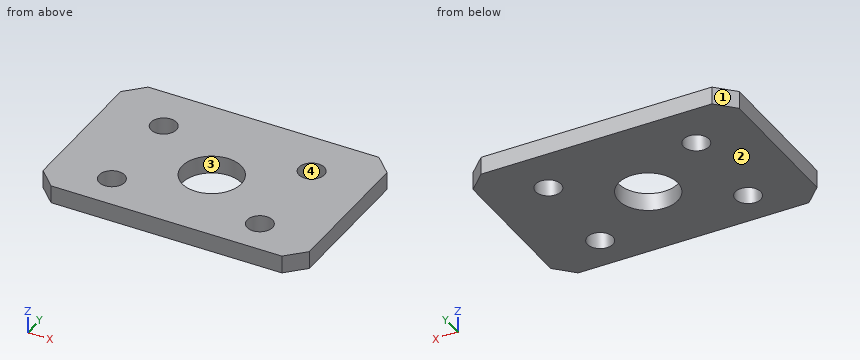
```python
from build123d import *

# Parameters (mm, degrees)
SKETCH_1_W               = 33
SKETCH_1_H               = 47
SKETCH_1_R               = 5
EXTRUDE_1_DEPTH          = 4
EXTRUDE_2_DEPTH          = 30
SKETCH_4_W               = 33
SKETCH_4_H               = 38
EXTRUDE_3_DEPTH          = 4
CHAMFER_1_SIZE           = 3
SKETCH_5_W               = 10
SKETCH_5_H               = 30
EXTRUDE_4_DEPTH          = 6
SKETCH_6_R               = 2.15
CUT_EXTRUDE_1_DEPTH      = 88.143559716
SKETCH_7_R               = 2.15
CUT_EXTRUDE_2_DEPTH      = 60
SKETCH_8_W               = 142.872393379
SKETCH_8_H               = 129.651084076
CUT_EXTRUDE_3_DEPTH      = 88.143559716
CUT_EXTRUDE_START        = -26
SKETCH_9_W               = 6
SKETCH_9_H               = 85
SKETCH_9_H_2             = 55
CUT_EXTRUDE_4_DEPTH      = 26
SKETCH_10_R              = 6.65
EXTRUDE_5_DEPTH          = 5.2
EXTRUDE_6_DEPTH          = 6
CHAMFER_2_SIZE           = 5.2
EXTRUDE_START            = -6
SKETCH_12_R              = 2.15
EXTRUDE_7_DEPTH          = 6
SKETCH_13_R              = 2.15
CUT_EXTRUDE_5_DEPTH      = 110.424128966
CUT_EXTRUDE_6_DEPTH      = 110.424128966
CUT_EXTRUDE_6_DEPTH_BACK = 110.424128966
SKETCH_14_W              = 45
SKETCH_14_H              = 81.938700875
SKETCH_15_W              = 48.923705392
SKETCH_15_H              = 34.943280138
CUT_EXTRUDE_7_DEPTH      = 6.2
CHAMFER_3_SIZE           = 3


with BuildPart() as part:
    # 草图1 → 凸台-拉伸1 (new body)
    with BuildSketch(Plane.XY):
        with Locations((16.5, 23.5)):
            Rectangle(SKETCH_1_W, SKETCH_1_H)
        with Locations((16.5, 31)):
            Circle(SKETCH_1_R, mode=Mode.SUBTRACT)
    extrude(amount=EXTRUDE_1_DEPTH)

    # 草图3 → 凸台-拉伸2 (add)
    with BuildSketch(Plane(origin=(0, 0, 0), x_dir=(-1, 0, 0), z_dir=(0, 0, -1))):
        Polygon((0, -38), (-33, -38), (-33, 47), (-39, 47), (-39, -63), (-26.75, -63), (-26.75, -43), (-6.25, -43), (-6.25, -63), (6, -63), (6, 47), (0, 47), align=None)
    extrude(amount=-EXTRUDE_2_DEPTH)

    # 草图4 → 凸台-拉伸3 (add)
    with BuildSketch(Plane(origin=(0, 0, 0), x_dir=(-1, 0, 0), z_dir=(0, 0, -1))):
        with Locations((-16.5, -19)):
            Rectangle(SKETCH_4_W, SKETCH_4_H)
    extrude(amount=-EXTRUDE_3_DEPTH)

    # 倒角1
    chamfer_1_edges = [part.edges().sort_by_distance(p)[0] for p in [
        (-6, 47, 15),
        (-6, -63, 15),
        (39, -63, 15),
        (39, 47, 15),
    ]]
    chamfer(chamfer_1_edges, length=CHAMFER_1_SIZE)

    # 草图5 → 凸台-拉伸4 (add)
    with BuildSketch(Plane(origin=(39, 0, 0), x_dir=(0, 0, -1), z_dir=(1, 0, 0))):
        with Locations((-35, -23)):
            Rectangle(SKETCH_5_W, SKETCH_5_H)
    extrude(amount=-EXTRUDE_4_DEPTH)

    # 草图6 → 切除-拉伸1 (cut, through all)
    with BuildSketch(Plane(origin=(39, 0, 0), x_dir=(0, 0, -1), z_dir=(1, 0, 0))):
        with Locations(Location((-11, -32, 0), (0, 0, 90))):
            Circle(SKETCH_6_R)
        with Locations(Location((-35, -32, 0), (0, 0, 90))):
            Circle(SKETCH_6_R)
        with Locations(Location((-11, -14, 0), (0, 0, 90))):
            Circle(SKETCH_6_R)
        with Locations(Location((-35, -14, 0), (0, 0, 90))):
            Circle(SKETCH_6_R)
    extrude(amount=-CUT_EXTRUDE_1_DEPTH, mode=Mode.SUBTRACT)

    # 草图7 → 切除-拉伸2 (cut)
    with BuildSketch(Plane.ZY.offset(6)):
        with Locations(Location((15, -53, 0), (0, 0, 270))):
            Circle(SKETCH_7_R)
    extrude(amount=-CUT_EXTRUDE_2_DEPTH, mode=Mode.SUBTRACT)

    # 镜向1: part across plane


with BuildPart() as part_1:
    add(part.part)
    add(part.part.mirror(Plane(origin=(39, 0, 0), x_dir=(0, 0, 1), z_dir=(1, 0, 0))))

    # 草图8 → 切除-拉伸3 (cut, through all)
    with BuildSketch(Plane(origin=(39, 0, 0), x_dir=(0, 0, -1), z_dir=(1, 0, 0))):
        with Locations((-14.281868294, -7.269848701)):
            Rectangle(SKETCH_8_W, SKETCH_8_H)
    extrude(amount=-CUT_EXTRUDE_3_DEPTH, mode=Mode.SUBTRACT)

    # 草图9 → 切除-拉伸4 (cut)
    with BuildSketch(Plane.XY.offset(30).offset(CUT_EXTRUDE_START)):
        with Locations((81, 4.5)):
            Rectangle(SKETCH_9_W, SKETCH_9_H)
        with Locations((42, 19.5)):
            Rectangle(SKETCH_9_W, SKETCH_9_H_2)
    extrude(amount=CUT_EXTRUDE_4_DEPTH, mode=Mode.SUBTRACT)

    # 草图10 → 凸台-拉伸5 (add)
    with BuildSketch(Plane.XY.offset(4)):
        Polygon((42, 47), (39, 44), (39, 17), (84, 17), (84, 44), (81, 47), align=None)
        with Locations((61.5, 31)):
            Circle(SKETCH_10_R, mode=Mode.SUBTRACT)
    extrude(amount=EXTRUDE_5_DEPTH)

    # 草图11 → 凸台-拉伸6 (add)
    with BuildSketch(Plane.ZY.offset(-39)):
        Polygon((40, -8), (4, -8), (4, 17), (9.2, 17), align=None)
    extrude(amount=-EXTRUDE_6_DEPTH)

    # 倒角2
    chamfer_2_edges = [part_1.edges().sort_by_distance(p)[0] for p in [
        (64.5, 17, 4),
    ]]
    chamfer(chamfer_2_edges, length=CHAMFER_2_SIZE - 0.0001)  # a hair under: the kernel refuses the full size

    # 草图12 → 凸台-拉伸7 (add)
    with BuildSketch(Plane(origin=(84, 0, 0), x_dir=(0, 0, -1), z_dir=(1, 0, 0)).offset(EXTRUDE_START)):
        Polygon((-30, -38), (-4, -38), (-4, -13), align=None)
        with Locations(Location((-11, -32, 0), (0, 0, 90))):
            Circle(SKETCH_12_R, mode=Mode.SUBTRACT)
    extrude(amount=EXTRUDE_7_DEPTH)

    # 草图13 → 切除-拉伸5 (cut, through all)
    with BuildSketch(Plane.XY.offset(9.2)):
        with Locations((49, 39)):
            Circle(SKETCH_13_R)
        with Locations((49, 23)):
            Circle(SKETCH_13_R)
        with Locations((74, 39)):
            Circle(SKETCH_13_R)
        with Locations((74, 23)):
            Circle(SKETCH_13_R)
    extrude(amount=-CUT_EXTRUDE_5_DEPTH, mode=Mode.SUBTRACT)

    # 草图14 → 切除-拉伸6 (cut, two sides: drawn at the far end of the back side and taken through both)
    with BuildSketch(Plane.XY.offset(9.2).offset(-CUT_EXTRUDE_6_DEPTH_BACK)):
        with Locations((61.5, -23.969350438)):
            Rectangle(SKETCH_14_W, SKETCH_14_H)
    extrude(amount=CUT_EXTRUDE_6_DEPTH + CUT_EXTRUDE_6_DEPTH_BACK, mode=Mode.SUBTRACT)

    # 草图15 → 切除-拉伸7 (cut)
    with BuildSketch(Plane.XY.offset(9.2)):
        with Locations((63.461852696, 34.471640069)):
            Rectangle(SKETCH_15_W, SKETCH_15_H)
    extrude(amount=-CUT_EXTRUDE_7_DEPTH, mode=Mode.SUBTRACT)

    # 倒角3
    chamfer_3_edges = [part_1.edges().sort_by_distance(p)[0] for p in [
        (84, 17, 1.5),
        (39, 17, 1.5),
    ]]
    chamfer(chamfer_3_edges, length=CHAMFER_3_SIZE)


solid = part_1.part
```
Source: CAD feature listing. Evaluate the final solid. Frame: model axes, mm. Face numbers are marked on the shaded views. Round coordinates to 2 decimals unless told otherwise and drop trailing zeros. Loops run counter-clockwise (first coordinate to the right, second up) from the corner with the lowest first, then second, coordinate; pieces in that order, holes last.
1. Section query B-B on y = 31. Output: boundary loops of the cut face in (x, z), and give its area (3 significant figures).
2. Ray query, L1, parallel to Y at x = 74, z = 1.2; L2, parallel to Y at x = 61.5, z = 2.5; L3, parallel to Y at x = 50, z = 1.05. Return the intervals inside material, ascending.
3. Section query A-A on z = 0.5. Output: boundary loops of the cut face in (x, y).
4. Section query C-C on x = 61.5. Output: boundary loops of the cut face in (y, z), and give its area (3 significant figures).
5. Mould query, pull axis Y, two halves, no side actions, for the marked faces 1, 2, 3 and 4. Classes: released by +Y, released by -Y, zero draft, split by the parting line, or undercut.
6. Section query D-D on x = 49. Output: boundary loops of the cut face in (y, z).
Answers below:
1. outline: (39, 0) - (56.5, 0) - (56.5, 3) - (39, 3) - close; (66.5, 0) - (84, 0) - (84, 3) - (66.5, 3) - close
1. area: 105 mm2
2. L1: y = 17 to 20.85, 25.15 to 36.85, 41.15 to 47
2. L2: y = 17 to 26, 36 to 47
2. L3: y = 17 to 21.1, 24.9 to 37.1, 40.9 to 47
3. outline: (39, 20) - (42, 17) - (81, 17) - (84, 20) - (84, 44) - (81, 47) - (42, 47) - (39, 44) - close; hole circle Ø4.3 at (49, 23); hole circle Ø4.3 at (49, 39); hole circle Ø10 at (61.5, 31); hole circle Ø4.3 at (74, 23); hole circle Ø4.3 at (74, 39)
4. outline: (17, 0) - (26, 0) - (26, 3) - (17, 3) - close; (36, 0) - (47, 0) - (47, 3) - (36, 3) - close
4. area: 60.0 mm2
5. face 1: released by +Y
5. face 2: zero draft
5. face 3: undercut
5. face 4: undercut
6. outline: (17, 0) - (20.85, 0) - (20.85, 3) - (17, 3) - close; (25.15, 0) - (36.85, 0) - (36.85, 3) - (25.15, 3) - close; (41.15, 0) - (47, 0) - (47, 3) - (41.15, 3) - close
